Print and shaded views of the part. All mm, measured from the part's lowest x, y and z. Round coordinates to 2 decimals unless told otherwise and drop trailing zeros. Order: outer loops, then holes, each group sorted by start corner. A loop starts at its lowest first (then second) coordinate and runs counter-clockwise, first axis right, second up. Notation, with made-up numbers: (54, 42) - (63, 42) arc R19 ccw to (63, 55) - close; hole circle Ø10 at (-26.75, -33). An arc over 180 degrees is marked (long way). Return JSON: item names as keys, results as strings. Group by question number.
Item 1: Saw through at C-C on y = 23.6. List the corners of the cut face in (x, z), and give its area (3 significant figures).
Item 2: Probe probe 1 along X at (y, z) = (23.5, 5.15); probe 2 along Y at (x, z) = (87.5, 3.75); probe 3 along X at (y, z) = (72, 1.6). List the from-to ranges inside material, lowest first.
Item 3: Saw through at B-B on x = 12. List the corners of the cut face in (y, z).
Item 4: Drop flat-ended pins along their axis: pin 1 (6 mm diameter, centred on x = 87.5, y = 23.6, fed in from +Z); pin 2 (3.5 mm diameter, centred on x = 86, y = 10, fed in from +Z); pin 3 (2 mm diameter, centred on x = 73, y = 62.5, fed in from +Z). Give the stop position or say it passes through.
Item 5: Saw through at A-A on y = 10. List the corners of the cut face in (x, z), and give its area (3 significant figures).
Item 6: Saw through at D-D on y = 72. List the corners of the cut face in (x, z).
Item 7: Two-plate mould, pull along Y, no slides. Class the marked faces 1 and 2: released by +Y, released by -Y, zero draft, split by the parting line, or undercut.
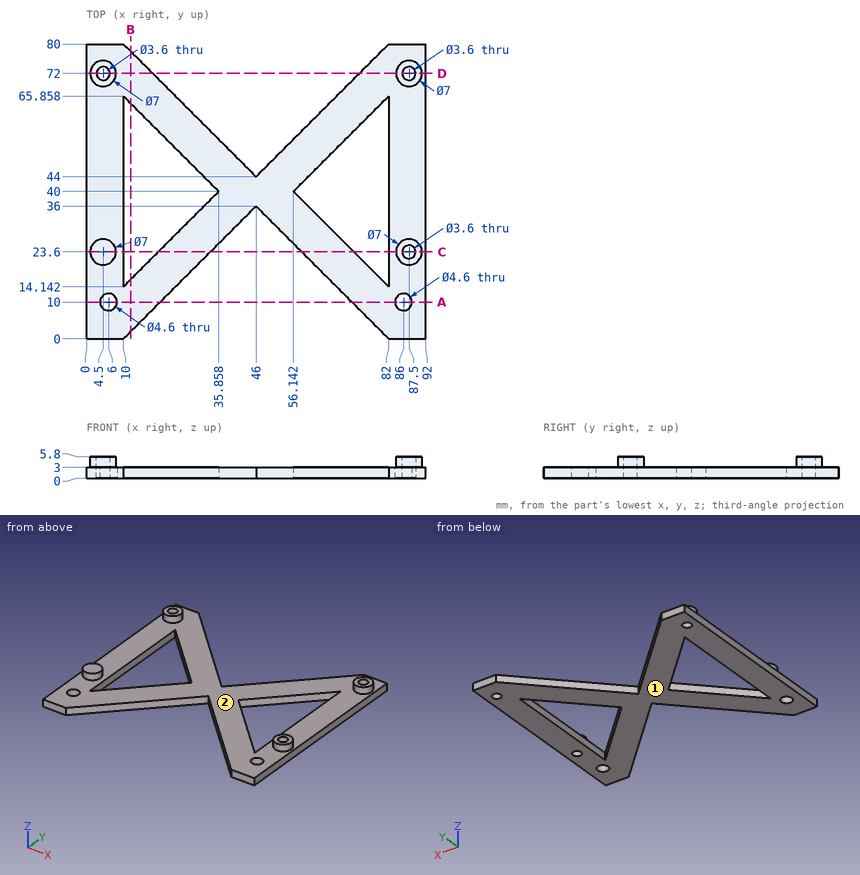
Filled in:
{
 "1": {"outline": "(0, 0) - (10, 0) - (10, 3) - (8, 3) - (8, 5.8) - (1, 5.8) - (1, 3) - (0, 3) - close; (19.46, 0) - (33.6, 0) - (33.6, 3) - (19.46, 3) - close; (58.4, 0) - (72.54, 0) - (72.54, 3) - (58.4, 3) - close; (82, 0) - (85.7, 0) - (85.7, 5.8) - (84, 5.8) - (84, 3) - (82, 3) - close; (89.3, 0) - (92, 0) - (92, 3) - (91, 3) - (91, 5.8) - (89.3, 5.8) - close", "area": "163 mm^2"},
 "2": {"probe 1": "x = 1 to 8, 84 to 85.7, 89.3 to 91", "probe 2": "y = 20.1 to 21.8, 25.4 to 27.1, 68.5 to 70.2, 73.8 to 75.5", "probe 3": "x = 0 to 2.7, 6.3 to 18, 74 to 85.7, 89.3 to 92"},
 "3": {"outline": "(2, 0) - (16.14, 0) - (16.14, 3) - (2, 3) - close; (63.86, 0) - (78, 0) - (78, 3) - (63.86, 3) - close"},
 "4": {"pin 1": "stops at z = 5.8", "pin 2": "passes through", "pin 3": "stops at z = 3"},
 "5": {"outline": "(0, 0) - (3.7, 0) - (3.7, 3) - (0, 3) - close; (8.3, 0) - (20, 0) - (20, 3) - (8.3, 3) - close; (72, 0) - (83.7, 0) - (83.7, 3) - (72, 3) - close; (88.3, 0) - (92, 0) - (92, 3) - (88.3, 3) - close", "area": "92.4 mm^2"},
 "6": {"outline": "(0, 0) - (2.7, 0) - (2.7, 5.8) - (1, 5.8) - (1, 3) - (0, 3) - close; (6.3, 0) - (18, 0) - (18, 3) - (8, 3) - (8, 5.8) - (6.3, 5.8) - close; (74, 0) - (85.7, 0) - (85.7, 5.8) - (84, 5.8) - (84, 3) - (74, 3) - close; (89.3, 0) - (92, 0) - (92, 3) - (91, 3) - (91, 5.8) - (89.3, 5.8) - close"},
 "7": {"face 1": "zero draft", "face 2": "undercut"}
}
